from build123d import *

# Parameters (mm, degrees)
F0_W     = 21.336
F0_H     = 11.43
F1_DEPTH = 22.1996
F2_W     = 15.24
F2_H     = 8.382
F3_DEPTH = 25.4
F4_W     = 3.048
F4_H     = 6.35
F5_DEPTH = 25.4
F6_R     = 3.048


with BuildPart() as f1:
    # F0 (on Front) → F1 (new body)
    with BuildSketch(Plane.XZ):
        Rectangle(F0_W, F0_H)
    extrude(amount=-F1_DEPTH)

    # F2 (on face) → F3 (cut)
    with BuildSketch(Plane.XZ):
        with Locations((0, 1.524)):
            Rectangle(F2_W, F2_H)
    extrude(amount=-F3_DEPTH, mode=Mode.SUBTRACT)

    # F4 (on face) → F5 (cut)
    with BuildSketch(Plane.XZ):
        with Locations((9.144, 2.54)):
            Rectangle(F4_W, F4_H)
    extrude(amount=-F5_DEPTH, mode=Mode.SUBTRACT)

    # F6
    f6_edges = [f1.edges().sort_by_distance(p)[0] for p in [
        (10.668, 11.0998, -5.715),
    ]]
    fillet(f6_edges, radius=F6_R)


solid = f1.part
Work out the finished part from the listing and answer in its coordinate system (mm). A direction names the side the tool comes from. Coordinates: 2 decimals unless noted, no trailing zeros. Loops run counter-clockwise (first coordinate to the right, second up) from the corner with the lowest first, then second, coordinate; pieces in that order, holes last. Notation, with made-up numbers: M 34.25,-20 L 84.25,-20 A17 cw 84.25,1 Z; hole C 77,-34.5 d11. An arc over 180 degrees is marked long. Answer in a Markdown table with one row per item. Add a question column.
1. A tool of negligible diameter and unlimited length cuts with its end or side. For faces 4 (the flat face through (0, 11, -2.667)), 5 (the flat face through (-9, 11, 5.715)), from which of +Z, -Z, +X, -X, +Y, -Y can it reach the whole face along a straight path? Write none if from no direction.
2. Find section B-B, the plane y = 4.25. Write down the section's boundary in (x, z) (3 decimals).
3. Find section A-A, the plane z = -1.5. Write down the section's boundary in (x, y), then the cut area to 3 significant figures.
4. Consider L1, parallel to X at y = 8.75, z = -2; L2, parallel to Z at x = -1.25, y = 16.25 (3 decimals); L3, parallel to X at y = 16.5, z = 3.5. Determine where each line is inside the solid, lowest interval first.
5. Find section C-C, the plane x = 5.75. Write down the section's boundary in (y, z) (3 decimals).
6. The mould has two halves that part along X. Classify faces 1 (the flat face through (10.668, 11, -2)), 2 (the flat face through (9, 11, -0.635)), 3 (the flat face through (7.62, 11, -2)): pulls with the +X half, pulls with the -X half, needs draft (parallel to the pull), parting line crosses it, or undercut.
7. Flat-ended cylindrical pins translate along their axes: P1, Ø1, axis at x = 4.5, y = 13.5, coming from the +Z side; P2, Ø1.5, axis at x = 9, y = 12.5, coming from the +Z side (3 decimals). Find the tip coordinate at first contact, or state that the pin passes through.
8. Find section D-D, the plane z = 1.75. Write down the section's boundary in (x, y), then the cut area to 3 significant figures.
Reported:
| question | item | result |
|---|---|---|
| 1 | face 4 | +Z, +Y, -Y |
| 1 | face 5 | +Z, +X, -X, +Y, -Y |
| 2 | outline | M -10.668,-5.715 L 7.62,-5.715 A3.048 ccw 10.668,-2.667 L 10.668,-0.635 L 7.62,-0.635 L 7.62,-2.667 L -7.62,-2.667 L -7.62,5.715 L -10.668,5.715 Z |
| 3 | outline | M -10.67,0 L -7.62,0 L -7.62,22.2 L -10.67,22.2 Z; M 7.62,0 L 10.67,0 L 10.67,22.2 L 7.62,22.2 Z |
| 3 | area | 135 mm^2 |
| 4 | L1 | x = -10.67 to -7.62, 7.62 to 10.67 |
| 4 | L2 | z = -5.715 to -2.667 |
| 4 | L3 | x = -10.67 to -7.62 |
| 5 | outline | M 0,-5.715 L 22.2,-5.715 L 22.2,-2.667 L 0,-2.667 Z |
| 6 | face 1 | pulls with the +X half |
| 6 | face 2 | needs draft |
| 6 | face 3 | undercut |
| 7 | P1 | stops at z = -2.67 |
| 7 | P2 | stops at z = -0.635 |
| 8 | outline | M -10.67,0 L -7.62,0 L -7.62,22.2 L -10.67,22.2 Z |
| 8 | area | 67.7 mm^2 |
